```python
from build123d import *

# Parameters (mm, degrees)
ESQUISSE1_R        = 1.925
ESQUISSE1_W        = 58
ESQUISSE1_H        = 20
BOSS_EXTRU_1_DEPTH = 5


with BuildPart() as part:
    # Esquisse1 → Boss.-Extru.1 (new body)
    with BuildSketch(Plane.XY):
        with BuildLine():
            Line((13.05, 32.5), (-13.05, 32.5))
            ThreePointArc((-13.05, 32.5), (-14.464213562, 31.914213562), (-15.05, 30.5))
            Line((-15.05, 30.5), (-15.05, 25))
            Line((-15.05, 25), (-13.55, 25))
            Line((-13.55, 25), (-13.55, 21))
            Line((-13.55, 21), (-20.45, 21))
            Line((-20.45, 21), (-20.45, 25))
            Line((-20.45, 25), (-18.95, 25))
            Line((-18.95, 25), (-18.95, 30.5))
            ThreePointArc((-18.95, 30.5), (-19.535786438, 31.914213562), (-20.95, 32.5))
            Line((-20.95, 32.5), (-23, 32.5))
            Line((-23, 32.5), (-23, 37.5))
            Line((-23, 37.5), (-25.999999067, 37.497633905))
            ThreePointArc((-25.999999067, 37.497633905), (-26.620839292, 37.398317642), (-27.180168114, 37.111163374))
            ThreePointArc((-27.180168114, 37.111163374), (-45.999999844, 0), (-27.180168114, -37.111163374))
            ThreePointArc((-27.180168114, -37.111163374), (-26.620839292, -37.398317642), (-25.999999067, -37.497633905))
            Line((-25.999999067, -37.497633905), (-23, -37.5))
            Line((-23, -37.5), (-23, -32.5))
            Line((-23, -32.5), (-20.95, -32.5))
            ThreePointArc((-20.95, -32.5), (-19.535786438, -31.914213562), (-18.95, -30.5))
            Line((-18.95, -30.5), (-18.95, -25))
            Line((-18.95, -25), (-20.45, -25))
            Line((-20.45, -25), (-20.45, -21))
            Line((-20.45, -21), (-13.55, -21))
            Line((-13.55, -21), (-13.55, -25))
            Line((-13.55, -25), (-15.05, -25))
            Line((-15.05, -25), (-15.05, -30.5))
            ThreePointArc((-15.05, -30.5), (-14.464213562, -31.914213562), (-13.05, -32.5))
            Line((-13.05, -32.5), (13.05, -32.5))
            ThreePointArc((13.05, -32.5), (14.464213562, -31.914213562), (15.05, -30.5))
            Line((15.05, -30.5), (15.05, -25))
            Line((15.05, -25), (13.55, -25))
            Line((13.55, -25), (13.55, -21))
            Line((13.55, -21), (20.45, -21))
            Line((20.45, -21), (20.45, -25))
            Line((20.45, -25), (18.95, -25))
            Line((18.95, -25), (18.95, -30.5))
            ThreePointArc((18.95, -30.5), (19.535786438, -31.914213562), (20.95, -32.5))
            Line((20.95, -32.5), (23, -32.5))
            Line((23, -32.5), (23, -37.5))
            Line((23, -37.5), (25.999999067, -37.497633905))
            ThreePointArc((25.999999067, -37.497633905), (26.620839292, -37.398317642), (27.180168114, -37.111163374))
            ThreePointArc((27.180168114, -37.111163374), (45.999999844, 0), (27.180168114, 37.111163374))
            ThreePointArc((27.180168114, 37.111163374), (26.620839292, 37.398317642), (25.999999067, 37.497633905))
            Line((25.999999067, 37.497633905), (23, 37.5))
            Line((23, 37.5), (23, 32.5))
            Line((23, 32.5), (20.95, 32.5))
            ThreePointArc((20.95, 32.5), (19.535786438, 31.914213562), (18.95, 30.5))
            Line((18.95, 30.5), (18.95, 25))
            Line((18.95, 25), (20.45, 25))
            Line((20.45, 25), (20.45, 21))
            Line((20.45, 21), (13.55, 21))
            Line((13.55, 21), (13.55, 25))
            Line((13.55, 25), (15.05, 25))
            Line((15.05, 25), (15.05, 30.5))
            ThreePointArc((15.05, 30.5), (14.464213562, 31.914213562), (13.05, 32.5))
        make_face()
        with Locations((27.75, 0)):
            Circle(ESQUISSE1_R, mode=Mode.SUBTRACT)
        with Locations((-21.933137835, -17)):
            Circle(ESQUISSE1_R, mode=Mode.SUBTRACT)
        with Locations((-21.933137835, 17)):
            Circle(ESQUISSE1_R, mode=Mode.SUBTRACT)
        with Locations((-10, 0)):
            Rectangle(ESQUISSE1_W, ESQUISSE1_H, mode=Mode.SUBTRACT)
    extrude(amount=BOSS_EXTRU_1_DEPTH)


solid = part.part
```
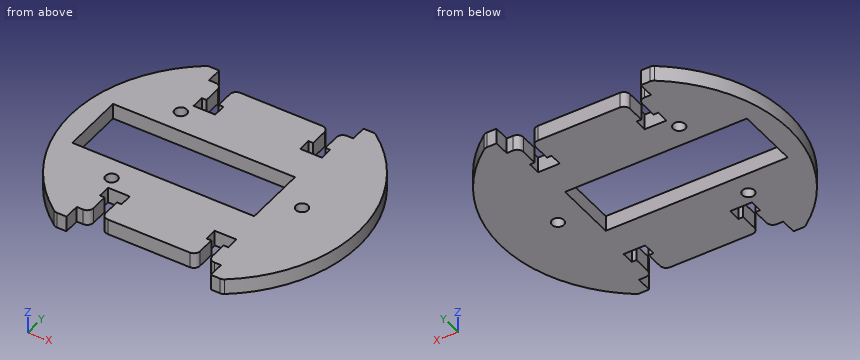
Build history of the part. All positions in model axes, mm. Round coordinates to 2 decimals unless told otherwise and drop trailing zeros. Loops run counter-clockwise (first coordinate to the right, second up) from the corner with the lowest first, then second, coordinate; pieces in that order, holes last.
Item 1: Saw through at A-A (x = -7). List the corners of the cut face in (y, z), then the cut area to 3 significant figures.
Item 2: Saw through at C-C (y = 17). List the corners of the cut face in (x, z), then the cut area to 3 significant figures.
Item 3: Saw through at D-D (z = 0.8). State how many separate pieces and enclosed holes the cut face has, then the cut area to 3 significant figures.
Item 4: Drill centre lines: line 1 along Y through (x, z) = (-3, 0.9); line 2 along X through (y, z) = (-1.5, 4.25); line 3 along X through (y, z) = (-23.5, 0.75). Where is each one in solid material? Low to high.
Item 5: Saw through at B-B (y = 0). List the corners of the cut face in (x, z) (3 decimals), then the cut area to 3 significant figures.
Item 6: Pin check, flat tips, straight feed: P1, Ø2, axis at y = 16, z = 1.5, coming from the +X side; P2, Ø1.6, axis at x = 14.5, z = 1.5, coming from the +Y side; P3, Ø2.5, axis at y = 28.5, z = 2.5, coming from the -X side. Stop position of each tip, or through.
Worked answers:
1. outline: (-32.5, 0) - (-10, 0) - (-10, 5) - (-32.5, 5) - close; (10, 0) - (32.5, 0) - (32.5, 5) - (10, 5) - close
1. area: 225 mm2
2. outline: (-42.74, 0) - (-23.86, 0) - (-23.86, 5) - (-42.74, 5) - close; (-20.01, 0) - (42.74, 0) - (42.74, 5) - (-20.01, 5) - close
2. area: 408 mm2
3. separate pieces: 1
3. enclosed holes: 4
3. area: 4,140 mm2
4. line 1: y = -32.5 to -10, 10 to 32.5
4. line 2: x = -45.98 to -39, 19 to 26.54, 28.96 to 45.98
4. line 3: x = -39.54 to -20.45, -13.55 to 13.55, 20.45 to 39.54
5. outline: (-46, 0) - (-39, 0) - (-39, 5) - (-46, 5) - close; (19, 0) - (25.825, 0) - (25.825, 5) - (19, 5) - close; (29.675, 0) - (46, 0) - (46, 5) - (29.675, 5) - close
5. area: 151 mm2
6. P1: stops at x = 43.49
6. P2: stops at y = 32.39
6. P3: stops at x = -37.06
